Job drawing, mm, ordinate dimensions from the low corner. One solid piece. A direction names the side the tool comes from. Coordinates: 2 decimals unless noted, no trailing zeros. Order: outer loops, then holes, each group sorted by start corner. A loop starts at its lowest first (then second) coordinate and runs counter-clockwise, first axis right, second up. Notation, with made-up numbers: M 28,57 L 40,57 A26 ccw 40,90 Z; hole C -34,-12.75 d4. An arc over 180 degrees is marked long. Write item = value, one per line. Start each with the question number.
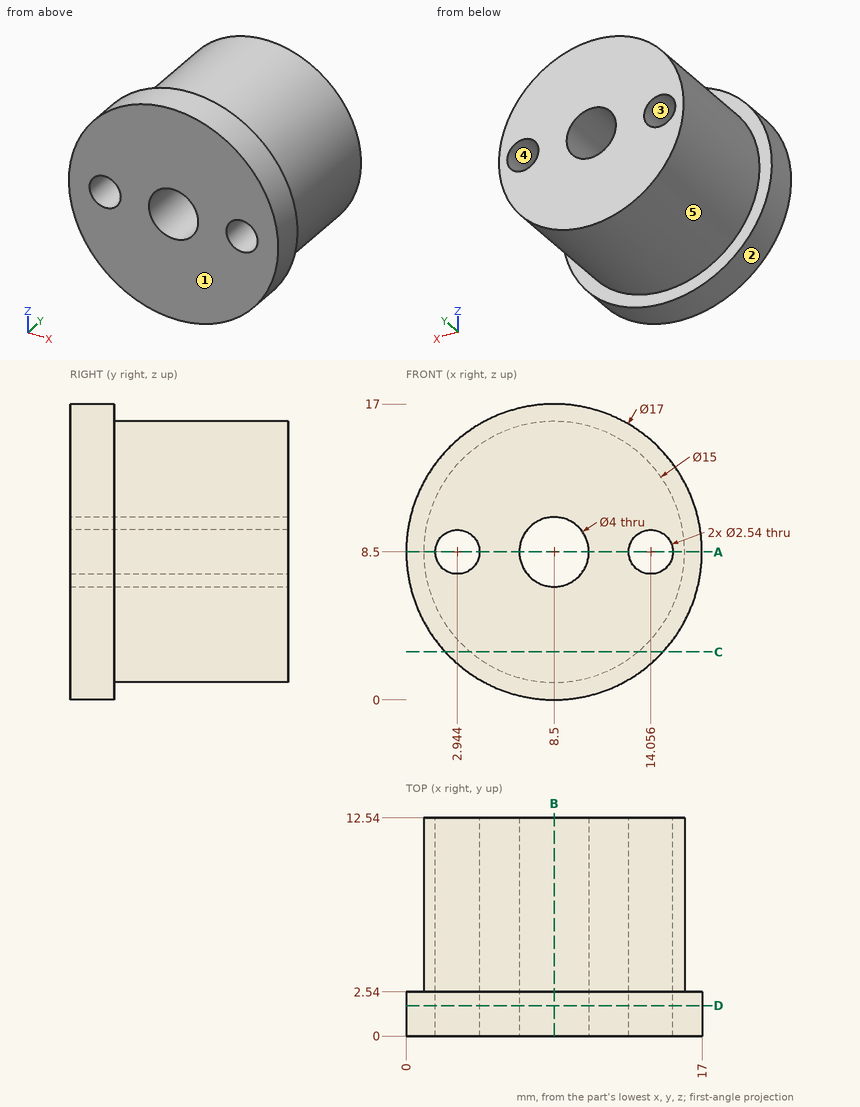
1. 3-axis set-ups, long thin cutter, end or side, ignore diameter. For the marked faces 4 and 5: which of +Z, -Z, +X, -X, +Y, -Y reach the whole face in a straight line?
2. Slice it at C-C (z = 2.75). Write the cut outline in (x, y) (1 decimal).
3. Slice it at D-D (y = 1.75). Write the cut outline in (x, z), plus the area to 3 significant figures.
4. Slice it at B-B (x = 8.5). Write the cut outline in (y, z), plus the area to 3 significant figures.
5. Slice it at A-A (z = 8.5). Write the cut outline in (x, y).
6. Flat gauge pins, fed straight in: pin 1 (6 mm diameter, centred on y = 10.5, z = 14.5, fed in from -X); pin 2 (5 mm diameter, centred on x = 2.5, y = 10, fed in from +Z); pin 3 (2 mm diameter, centred on y = 3, z = 2.5, fed in from +X). Where does each tip first touch, or does it go through?
7. Probe L1, parallel to X at y = 4.25, z = 8.5; L2, parallel to Z at x = 7, y = 1 (1 decimal); L3, parallel to Z at x = 3, y = 7. List the from-to ranges inside material, lowest first.
8. Mould opens along X. For the marked faces 1, 2 and 3 say: released by +X, released by -X, zero draft, split by the parting line, or undercut.
Calculated:
q1.face_4 = +Y, -Y
q1.face_5 = +Y
q2.outline = M 2.2,0 L 14.8,0 L 14.8,2.5 L 13.3,2.5 L 13.3,12.5 L 3.7,12.5 L 3.7,2.5 L 2.2,2.5 Z
q3.outline = C 8.5,8.5 d17; hole C 2.94,8.5 d2.54; hole C 8.5,8.5 d4; hole C 14.06,8.5 d2.54
q3.area = 204 mm²
q4.outline = M 0,0 L 2.54,0 L 2.54,1 L 12.54,1 L 12.54,6.5 L 0,6.5 Z; M 0,10.5 L 12.54,10.5 L 12.54,16 L 2.54,16 L 2.54,17 L 0,17 Z
q4.area = 143 mm²
q5.outline = M 0,0 L 1.67,0 L 1.67,12.54 L 1,12.54 L 1,2.54 L 0,2.54 Z; M 4.21,0 L 6.5,0 L 6.5,12.54 L 4.21,12.54 Z; M 10.5,0 L 12.79,0 L 12.79,12.54 L 10.5,12.54 Z; M 15.33,0 L 17,0 L 17,2.54 L 16,2.54 L 16,12.54 L 15.33,12.54 Z
q6.pin_1 = 1.63
q6.pin_2 = 15.13
q6.pin_3 = 15.29
q7.L1 = 1 to 1.67, 4.21 to 6.5, 10.5 to 12.79, 15.33 to 16
q7.L2 = 0.1 to 7.2, 9.8 to 16.9
q7.L3 = 3.4 to 7.23, 9.77 to 13.6
q8.face_1 = zero draft
q8.face_2 = split by the parting line
q8.face_3 = undercut
